Read the model definition and answer for the solid it produces. Units are mm, in the model's axes. Give positions to 0.01 mm unless a question says otherwise; leave off trailing zeros. Order: outer loops, then holes, each group sorted by start corner. A loop starts at its lowest first (then second) coordinate and runs counter-clockwise, first axis right, second up.
```python
from build123d import *

# Parameters (mm, degrees)
SKETCH1_W           = 200
SKETCH1_H           = 150
BOSS_EXTRUDE1_DEPTH = 6
SKETCH3_W           = 100
SKETCH3_H           = 97.5
CUT_EXTRUDE1_DEPTH  = 6
BOSS_EXTRUDE3_DEPTH = 6
SKETCH5_W           = 6
SKETCH5_H           = 15
CUT_EXTRUDE2_DEPTH  = 6


with BuildPart() as part:
    # Sketch1 → Boss-Extrude1 (new body)
    with BuildSketch(Plane.XY):
        with Locations((-100, 75)):
            Rectangle(SKETCH1_W, SKETCH1_H)
        with BuildLine():
            Line((-175, 110), (-175, 125))
            Line((-175, 125), (-25, 125))
            Line((-25, 125), (-25, 110))
            ThreePointArc((-25, 110), (-30.691670032, 81.340701386), (-46.902810588, 57.03125))
            ThreePointArc((-46.902810588, 57.03125), (-100, 27.5), (-153.097189412, 57.03125))
            ThreePointArc((-153.097189412, 57.03125), (-169.308329968, 81.340701386), (-175, 110))
        make_face(mode=Mode.SUBTRACT)
    extrude(amount=BOSS_EXTRUDE1_DEPTH)

    # Sketch3 → Cut-Extrude1 (cut)
    with BuildSketch(Plane.XY.offset(6)):
        with Locations((-150, 76.25)):
            Rectangle(SKETCH3_W, SKETCH3_H)
    extrude(amount=-CUT_EXTRUDE1_DEPTH, mode=Mode.SUBTRACT)

    # Sketch4 → Boss-Extrude3 (add)
    with BuildSketch(Plane.XY.offset(6)):
        with BuildLine():
            Line((-200, 27.5), (-250, 27.5))
            ThreePointArc((-250, 27.5), (-280.378472024, 35.379505335), (-303.097189412, 57.03125))
            ThreePointArc((-303.097189412, 57.03125), (-319.308329968, 81.340701386), (-325, 110))
            Line((-325, 110), (-325, 125))
            Line((-325, 125), (-200, 125))
            Line((-200, 125), (-200, 150))
            Line((-200, 150), (-350, 150))
            Line((-350, 150), (-350, 0))
            Line((-350, 0), (-200, 0))
            Line((-200, 0), (-200, 27.5))
        make_face()
    extrude(amount=-BOSS_EXTRUDE3_DEPTH)

    # Sketch5 → Cut-Extrude2 (cut)
    with BuildSketch(Plane.XY.offset(6)):
        with Locations((-175, 142.5)):
            Rectangle(SKETCH5_W, SKETCH5_H)
        with Locations((-175, 20)):
            Rectangle(SKETCH5_W, SKETCH5_H)
    extrude(amount=-CUT_EXTRUDE2_DEPTH, mode=Mode.SUBTRACT)


solid = part.part
```
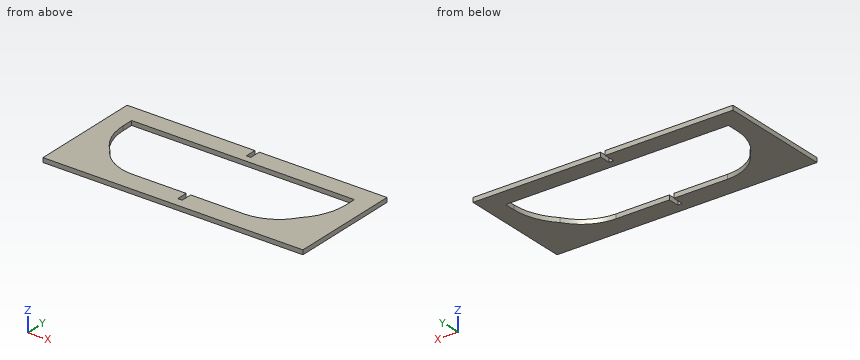
1) The part is cut by section C-C on z = 1.1. Determine the outline of the cut face in (x, y), and give its area (3 significant figures).
Final values:
outline: (-350, 0) - (0, 0) - (0, 150) - (-172, 150) - (-172, 135) - (-178, 135) - (-178, 150) - (-350, 150) - close; hole (-325, 110) arc R75 ccw to (-303.1, 57.03) arc R62.5 ccw to (-250, 27.5) - (-178, 27.5) - (-178, 12.5) - (-172, 12.5) - (-172, 27.5) - (-100, 27.5) arc R62.5 ccw to (-46.9, 57.03) arc R75 ccw to (-25, 110) - (-25, 125) - (-325, 125) - close
area: 26,000 mm2
2) Consider L1, parallel to Y at x = -220.5, z = 3.4; L2, parallel to X at y = 20.5, z = 2.25; L3, parallel to X at y = 109.5, z = 0.3. Determine where each line is inside the solid, lowest interval first.
Final values:
L1: y = 0 to 27.5, 125 to 150
L2: x = -350 to -178, -172 to 0
L3: x = -350 to -325, -25 to 0
3) Given pin 1 (3 mm diameter, centred on y = 18.5, z = 3, fed in from +X), flat-ended and moving along its own axis, determine where the tip first touches the part or whether it passes through.
Final values:
pin 1: stops at x = 0
4) The part is cut by section B-B on x = -155. Determine the outline of the cut face in (y, z), and give its area (3 significant figures).
Final values:
outline: (0, 0) - (27.5, 0) - (27.5, 6) - (0, 6) - close; (125, 0) - (150, 0) - (150, 6) - (125, 6) - close
area: 315 mm2
5) The part is cut by section A-A on y = 22.5. Determine the outline of the cut face in (x, z).
Final values:
outline: (-350, 0) - (-178, 0) - (-178, 6) - (-350, 6) - close; (-172, 0) - (0, 0) - (0, 6) - (-172, 6) - close
